from build123d import *

# Parameters (mm, degrees)
SKETCH2_W                                           = 98.778145
SKETCH2_H                                           = 68.778145
BOSS_EXTRUDE1_DEPTH                                 = 3.5
FILLET1_R                                           = 1
FILLET2_R                                           = 2.5
CUT_EXTRUDE1_DEPTH                                  = 1.5
CSK_FOR_M3_COUNTERSUNK_FLAT_HEAD_SCREW1_D           = 3.4
CSK_FOR_M3_COUNTERSUNK_FLAT_HEAD_SCREW1_DEPTH       = 10
CSK_FOR_M3_COUNTERSUNK_FLAT_HEAD_SCREW1_CSINK_D     = 6.3
CSK_FOR_M3_COUNTERSUNK_FLAT_HEAD_SCREW1_CSINK_ANGLE = 90
CSK_FOR_M3_COUNTERSUNK_FLAT_HEAD_SCREW1_TIP         = 1.021463052


with BuildPart() as part:
    # Sketch2 → Boss-Extrude1 (new body)
    with BuildSketch(Plane(origin=(0, 0, 0), x_dir=(1, 0, 0), z_dir=(0, 1, 0))):
        Rectangle(SKETCH2_W, SKETCH2_H)
    extrude(amount=BOSS_EXTRUDE1_DEPTH)

    # Fillet1
    fillet1_edges = [part.edges().sort_by_distance(p)[0] for p in [
        (49.3890725, 3.5, 0),
        (0, 3.5, -34.3890725),
        (-49.3890725, 3.5, 0),
        (0, 3.5, 34.3890725),
    ]]
    fillet(fillet1_edges, radius=FILLET1_R)

    # Fillet2
    # the kernel refuses this fillet: 2.5 mm, written as the material it takes off along each edge
    with BuildSketch(Plane(origin=(46.8890725, 3.5, 31.8890725), x_dir=(0, 0, 1), z_dir=(-1, 0, 0))) as fillet2_piece_1:
        with BuildLine():
            CenterArc((1.5, -1), 1, 0, 90)
            Line((2.5, -1), (2.5, 0))
            Line((2.5, 0), (1.5, 0))
        make_face()
    revolve(axis=Axis((46.8890725, 3.5, 31.8890725), (0, 1, 0)), revolution_arc=90, mode=Mode.SUBTRACT)
    with BuildSketch(Plane(origin=(-46.8890725, 3.5, 31.8890725), x_dir=(-1, 0, 0), z_dir=(0, 0, -1))) as fillet2_piece_2:
        with BuildLine():
            CenterArc((1.5, -1), 1, 0, 90)
            Line((2.5, -1), (2.5, 0))
            Line((2.5, 0), (1.5, 0))
        make_face()
    revolve(axis=Axis((-46.8890725, 3.5, 31.8890725), (0, 1, 0)), revolution_arc=90, mode=Mode.SUBTRACT)
    with BuildSketch(Plane(origin=(46.8890725, 3.5, -31.8890725), x_dir=(1, 0, 0), z_dir=(0, 0, 1))) as fillet2_piece_3:
        with BuildLine():
            CenterArc((1.5, -1), 1, 0, 90)
            Line((2.5, -1), (2.5, 0))
            Line((2.5, 0), (1.5, 0))
        make_face()
    revolve(axis=Axis((46.8890725, 3.5, -31.8890725), (0, 1, 0)), revolution_arc=90, mode=Mode.SUBTRACT)
    with BuildSketch(Plane(origin=(-46.8890725, 3.5, -31.8890725), x_dir=(0, 0, -1), z_dir=(1, 0, 0))) as fillet2_piece_4:
        with BuildLine():
            CenterArc((1.5, -1), 1, 0, 90)
            Line((2.5, -1), (2.5, 0))
            Line((2.5, 0), (1.5, 0))
        make_face()
    revolve(axis=Axis((-46.8890725, 3.5, -31.8890725), (0, 1, 0)), revolution_arc=90, mode=Mode.SUBTRACT)
    with BuildSketch(Plane(origin=(-49.3890725, -6.25, -34.3890725), x_dir=(0, 0, 1), z_dir=(0, 1, 0)), Plane(origin=(-49.3890725, -6.25, 34.3890725), x_dir=(1, 0, 0), z_dir=(0, 1, 0))) as fillet2_piece_5:
        with BuildLine():
            CenterArc((FILLET2_R, FILLET2_R), FILLET2_R, 180, 90)
            Line((0, FILLET2_R), (0, 0))
            Line((0, 0), (FILLET2_R, 0))
        make_face()
    extrude(amount=9.75, mode=Mode.SUBTRACT)
    with BuildSketch(Plane(origin=(49.3890725, -6.25, -34.3890725), x_dir=(0, 0, 1), z_dir=(0, 1, 0)), Plane(origin=(49.3890725, -6.25, 34.3890725), x_dir=(-1, 0, 0), z_dir=(0, 1, 0))) as fillet2_piece_6:
        with BuildLine():
            CenterArc((FILLET2_R, -FILLET2_R), FILLET2_R, 90, 90)
            Line((0, -FILLET2_R), (0, 0))
            Line((0, 0), (FILLET2_R, 0))
        make_face()
    extrude(amount=9.75, mode=Mode.SUBTRACT)

    # Sketch3 → Cut-Extrude1 (cut)
    with BuildSketch(Plane.XZ):
        with BuildLine():
            Line((47.8890725, -31.8890725), (47.8890725, 31.8890725))
            ThreePointArc((47.8890725, 31.8890725), (47.596179281, 32.596179281), (46.8890725, 32.8890725))
            Line((46.8890725, 32.8890725), (-46.8890725, 32.8890725))
            ThreePointArc((-46.8890725, 32.8890725), (-47.596179281, 32.596179281), (-47.8890725, 31.8890725))
            Line((-47.8890725, 31.8890725), (-47.8890725, -31.8890725))
            ThreePointArc((-47.8890725, -31.8890725), (-47.596179281, -32.596179281), (-46.8890725, -32.8890725))
            Line((-46.8890725, -32.8890725), (46.8890725, -32.8890725))
            ThreePointArc((46.8890725, -32.8890725), (47.596179281, -32.596179281), (47.8890725, -31.8890725))
        make_face()
    extrude(amount=-CUT_EXTRUDE1_DEPTH, mode=Mode.SUBTRACT)

    # CSK for M3 Countersunk Flat Head Screw1
    with Locations(Plane(origin=(-40.911963263, 3.5, -25.911963263), x_dir=(0, 0, 1), z_dir=(0, 1, 0))):
        with Locations((0, 0), (0, 81.823926071), (51.823926071, 81.823926071), (51.823926071, 0)):
            CounterSinkHole(CSK_FOR_M3_COUNTERSUNK_FLAT_HEAD_SCREW1_D / 2, CSK_FOR_M3_COUNTERSUNK_FLAT_HEAD_SCREW1_CSINK_D / 2, depth=CSK_FOR_M3_COUNTERSUNK_FLAT_HEAD_SCREW1_DEPTH, counter_sink_angle=CSK_FOR_M3_COUNTERSUNK_FLAT_HEAD_SCREW1_CSINK_ANGLE)
            with Locations((0, 0, -(CSK_FOR_M3_COUNTERSUNK_FLAT_HEAD_SCREW1_DEPTH + CSK_FOR_M3_COUNTERSUNK_FLAT_HEAD_SCREW1_TIP / 2))):  # 118° drill point
                Cone(0, CSK_FOR_M3_COUNTERSUNK_FLAT_HEAD_SCREW1_D / 2, CSK_FOR_M3_COUNTERSUNK_FLAT_HEAD_SCREW1_TIP, mode=Mode.SUBTRACT)


solid = part.part
CAD build for the part. Positions are in the model's coordinates, mm. A direction names the side the tool comes from. Give positions to 0.01 mm unless a question says otherwise; leave off trailing zeros. Loops run counter-clockwise (first coordinate to the right, second up) from the corner with the lowest first, then second, coordinate; pieces in that order, holes last. Notation, with made-up numbers: M 48.25,89 L 66.25,89 A9 cw 66.25,97 Z; hole C 31,84 d8. An arc over 180 degrees is marked long. One line per question, with ' | ' between items. Start each with the question number.
1. 3-axis set-ups, long thin cutter, end or side, ignore diameter. For faces 1 (the face through (-1, 1.5, 0)), 2 (the face through (-49.389, 1, 0)): which of +Z, -Z, +X, -X, +Y, -Y reach the whole face in a straight line?
2. Two-plate mould, pull along X, no slides. Class faces 3 (the face through (48.637, 1.232, 33.676)), 4 (the face through (-48.637, 1.232, -33.676)), 5 (the face through (-1, 3.5, 0)), 6 (the face through (-39.76, 1.77, -24.66)): pulls with the +X half, pulls with the -X half, needs draft (parallel to the pull), parting line crosses it, or undercut.
3. Saw through at B-B on z = -7. Give the cut face in (x, y).
4. Saw through at A-A on y = 0.95. Give the cut face in (x, z), plus the area to 3 significant figures.
5. Flat gauge pins, fed straight in: pin 1 (5.5 mm diameter, centred on x = 40.91, z = 25.91, fed in from -Y); pin 2 (3 mm diameter, centred on x = 40.91, z = -25.91, fed in from -Y). Where does each tip first touch, or does it go through?
6. Saw through at C-C on x = -23. Give the cut face in (y, z), plus the area to 3 significant figures.
7. Probe L1, parallel to Z at x = -42.5, y = 0.45; L2, parallel to X at y = 1.1, z = 11; L3, parallel to X at y = 2.8, z = -26. List the from-to ranges inside material, lowest first. Write a range as from..to.
Result sheet:
1) face 1: -Y | face 2: +Z, -Z, -X, +Y, -Y
2) face 3: pulls with the +X half | face 4: pulls with the -X half | face 5: needs draft | face 6: undercut
3) outline: M -49.39,0 L -47.89,0 L -47.89,1.5 L 47.89,1.5 L 47.89,0 L 49.39,0 L 49.39,2.5 A1 ccw 48.39,3.5 L -48.39,3.5 A1 ccw -49.39,2.5 Z
4) outline: M -49.39,-31.89 A2.5 ccw -46.89,-34.39 L 46.89,-34.39 A2.5 ccw 49.39,-31.89 L 49.39,31.89 A2.5 ccw 46.89,34.39 L -46.89,34.39 A2.5 ccw -49.39,31.89 Z; hole M -47.89,-31.89 A1 ccw -46.89,-32.89 L 46.89,-32.89 A1 ccw 47.89,-31.89 L 47.89,31.89 A1 ccw 46.89,32.89 L -46.89,32.89 A1 ccw -47.89,31.89 Z | area: 489 mm^2
5) pin 1: stops at y = 1.5 | pin 2: passes through
6) outline: M 0,-34.39 L 2.5,-34.39 A1 ccw 3.5,-33.39 L 3.5,33.39 A1 ccw 2.5,34.39 L 0,34.39 L 0,32.89 L 1.5,32.89 L 1.5,-32.89 L 0,-32.89 Z | area: 142 mm^2
7) L1: z = -34.39..-32.89, 32.89..34.39 | L2: x = -49.39..-47.89, 47.89..49.39 | L3: x = -49.34..-43.36, -38.46..38.46, 43.36..49.34
